Could you check a few things on this drawing? It's one solid part, dimensions in mm from its lowest x, y, z. Coordinates: 2 decimals unless noted, no trailing zeros. Order: outer loops, then holes, each group sorted by start corner. A loop starts at its lowest first (then second) coordinate and runs counter-clockwise, first axis right, second up. Notation, with made-up numbers: (66.5, 68) - (90.5, 68) arc R23 cw to (90.5, 84) - close; hole circle Ø5 at (15.5, -18.5). An arc over 180 degrees is marked (long way). Return JSON: item names as keys, results as strings. Group by question number.
1) Imagine slicing it at A-A (z = 574). Write out the boundary of the cut face in (x, y), and give its area (3 significant figures).
2) For pin 1 Ø12 at (y, z) = (63.5, 134) entering from +X; pin 2 Ø3 at (x, y) = (1185.5, 58.5) entering from +Z; pin 3 Ø16 at (x, z) = (20, 26.5) entering from -Y; pin 4 Ø10 at (y, z) = (29.5, 275) entering from -X, each with a flat end and sliding along its axis, tell me the tip position at first contact or that it passes through.
3) If we mould it in two halves opening along X, with no side actions, what happens to the marked faces 1 and 2? For each: pulls with the +X half, pulls with the -X half, needs draft (parallel to the pull), parting line crosses it, or undercut.
4) Imagine slicing it at B-B (x = 1578.5). Write out the boundary of the cut face in (y, z), and give its area (3 significant figures).
5) If I drill on line 1 along Z through (x, y) = (20, 37); line 2 along X through (y, z) = (53, 623); line 3 along X through (y, z) = (68, 376), over which ranges is the centre line in solid material (lowest first)?
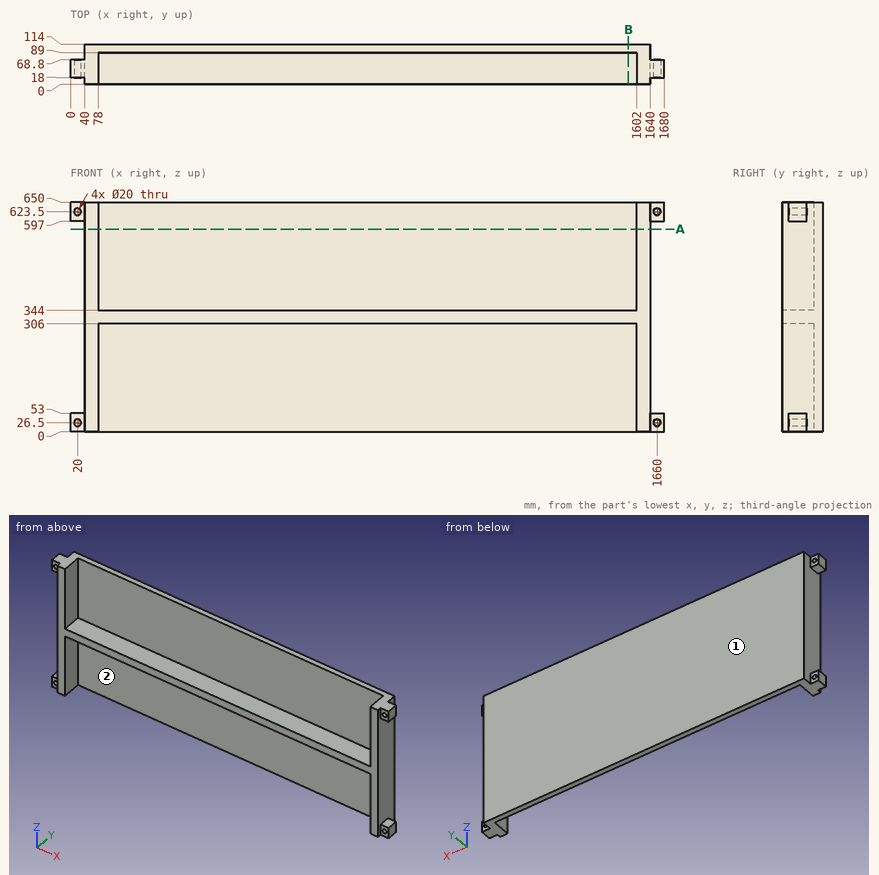
Calculated:
{
 "1": {"outline": "(40, 0) - (78, 0) - (78, 89) - (1602, 89) - (1602, 0) - (1640, 0) - (1640, 114) - (40, 114) - close", "area": "46,800 mm2"},
 "2": {"pin 1": "x = 1640", "pin 2": "z = 344", "pin 3": "through", "pin 4": "x = 40"},
 "3": {"face 1": "needs draft", "face 2": "undercut"},
 "4": {"outline": "(0, 306) - (89, 306) - (89, 0) - (114, 0) - (114, 650) - (89, 650) - (89, 344) - (0, 344) - close", "area": "19,600 mm2"},
 "5": {"line 1": "0 to 16.5, 36.5 to 53, 597 to 613.5, 633.5 to 650", "line 2": "0 to 10.01, 29.99 to 78, 1602 to 1650.01, 1669.99 to 1680", "line 3": "40 to 78, 1602 to 1640"}
}
